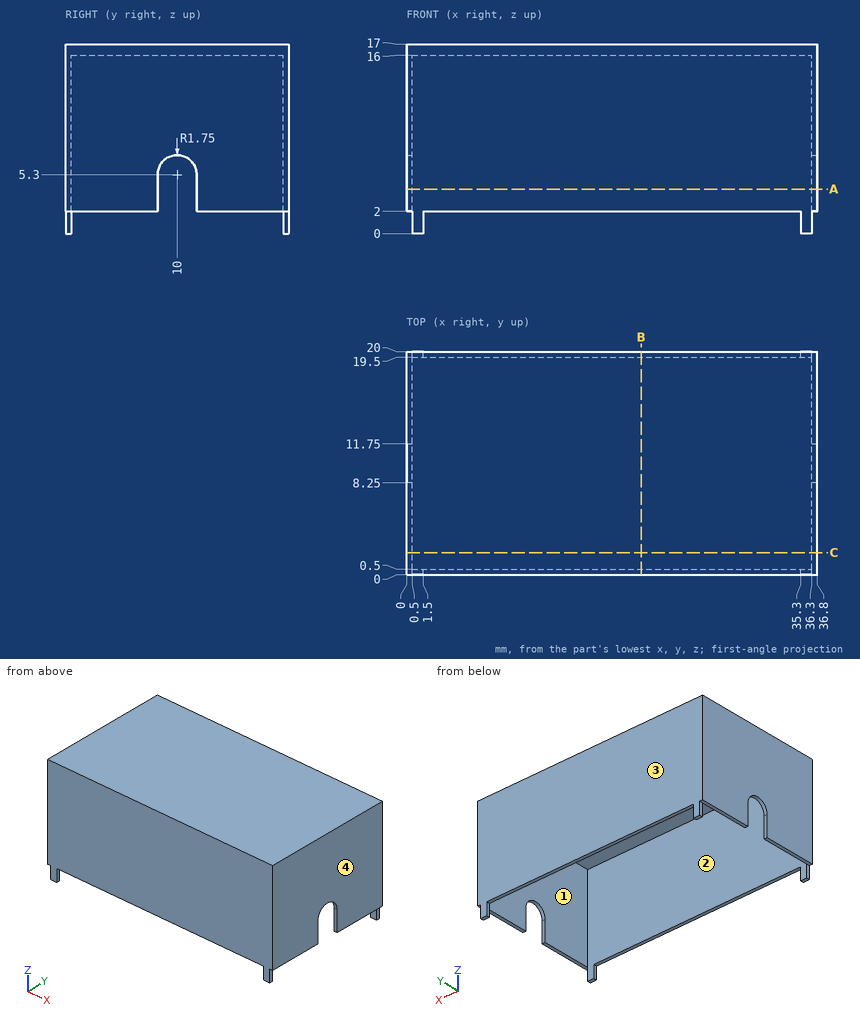
Here's the drawing with two shaded views (mm, measured from the low corner). I have some questions. Give positions to 0.01 mm unless a question says otherwise; leave off trailing zeros. Loops run counter-clockwise (first coordinate to the right, second up) from the corner with the lowest first, then second, coordinate; pieces in that order, holes last. Notation, with made-up numbers: (46.25, 62.25) - (82.25, 62.25) arc R8 ccw to (82.25, 77.25) - close; hole circle Ø1 at (-19, -16). An arc over 180 degrees is marked (long way). Return JSON: item names as keys, results as strings.
1. I'm going to push flat-ended pins straight in: pin 1 Ø6 at (y, z) = (14.5, 12.5) entering from -X; pin 2 Ø0.6 at (y, z) = (0.5, 0.5) entering from -X; pin 3 Ø9.5 at (x, y) = (10.5, 13) entering from -Z. Where does each tip first touch, or does it pass through?
Output values:
{"pin 1": "stops at x = 0", "pin 2": "stops at x = 0.5", "pin 3": "stops at z = 16"}
2. If I drill on line 1 (X direction, y = 8, z = 12); line 2 (Y direction, x = 3.5, z = 11); line 3 (Z direction, x = 13.5, y = 4), over which ranges is the centre line in solid material (lowest first)?
Output values:
{"line 1": "x = 0 to 0.5, 36.3 to 36.8", "line 2": "y = 0 to 0.5, 19.5 to 20", "line 3": "z = 16 to 17"}
3. We'd pull the mould along Y, two halves only. Please class the marked faces 1, 2, 3 and 4: +Y half, -Y half, draft (parallel to the pull), parting line (faces both ways), or undercut.
Output values:
{"face 1": "undercut", "face 2": "undercut", "face 3": "+Y half", "face 4": "draft"}
4. I want a section at A-A on z = 4. Please give me the cut outline in (x, y).
Output values:
{"outline": "(0, 0) - (36.8, 0) - (36.8, 8.25) - (36.3, 8.25) - (36.3, 0.5) - (0.5, 0.5) - (0.5, 8.25) - (0, 8.25) - close; (0, 11.75) - (0.5, 11.75) - (0.5, 19.5) - (36.3, 19.5) - (36.3, 11.75) - (36.8, 11.75) - (36.8, 20) - (0, 20) - close"}
5. I want a section at B-B on x = 21. Please give me the cut outline in (y, z).
Output values:
{"outline": "(0, 2) - (0.5, 2) - (0.5, 16) - (19.5, 16) - (19.5, 2) - (20, 2) - (20, 17) - (0, 17) - close"}
6. I want a section at C-C on y = 2. Please give me the cut outline in (x, z).
Output values:
{"outline": "(0, 2) - (0.5, 2) - (0.5, 16) - (36.3, 16) - (36.3, 2) - (36.8, 2) - (36.8, 17) - (0, 17) - close"}
